The drawing under review shows one solid part. Ordinate dimensions are in mm from its lowest x, y, z. Give positions to 0.01 mm unless a question says otherwise; leave off trailing zeros. Loops run counter-clockwise (first coordinate to the right, second up) from the corner with the lowest first, then second, coordinate; pieces in that order, holes last. Notation, with made-up numbers: M 18,75.5 L 65,75.5 A18 cw 65,89.5 Z; hole C -13,-6.5 d4. An arc over 180 degrees is marked long. Write item = value, one per line. Start each with the question number.
1. For pin 1 (2 mm diameter, centred on y = 4, z = 7, fed in from -X), flat-tipped, find the tip position at first contact; note if it passes through.
2. We need section D-D on y = 4.2. Give the boundary of the cut face in (x, z).
3. Wall thickness on line 1 along Z through (x, y) = (80, 2.55); line 2 along X through (y, z) = (3.05, 10); line 3 along Z through (x, y) = (49, 2.35): over which ranges is each line inside the solid? List them lowest first. Write a range as from..to.
4. We need section A-A on x = 50. Give the boundary of the cut face in (y, z).
5. We need section B-B on z = 13.8. Give the boundary of the cut face in (x, y), then the cut area to 3 significant figures.
6. We need section C-C on x = 25. Give the boundary of the cut face in (y, z).
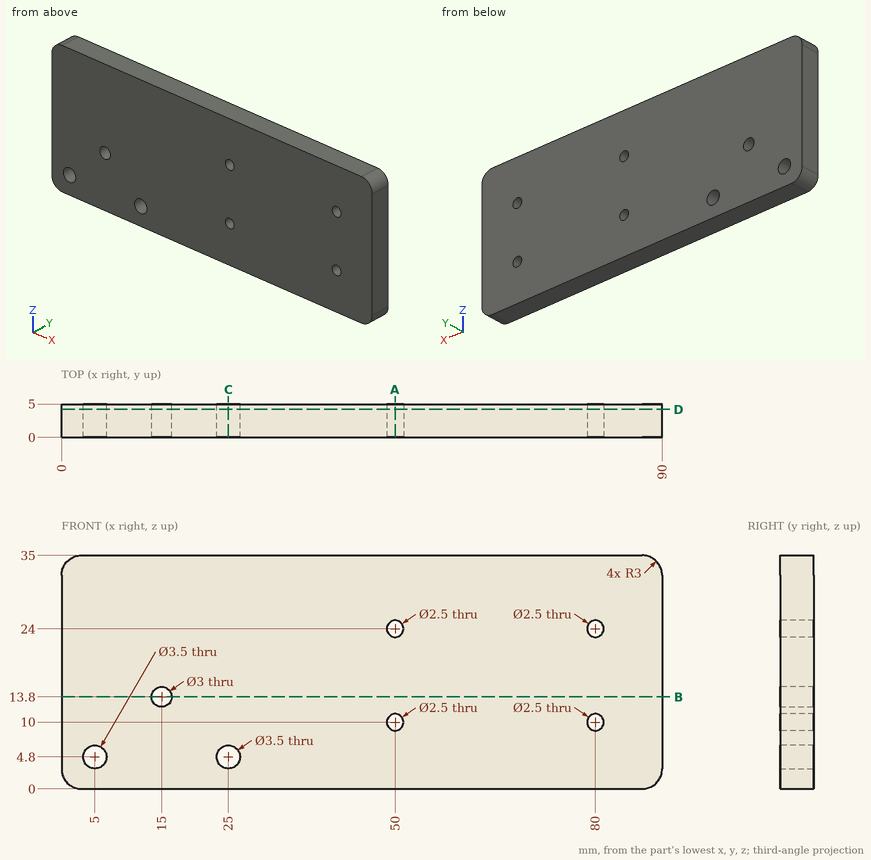
Final values:
q1.pin_1 = 0
q2.outline = M 0,3 A3 ccw 3,0 L 87,0 A3 ccw 90,3 L 90,32 A3 ccw 87,35 L 3,35 A3 ccw 0,32 Z; hole C 5,4.8 d3.5; hole C 15,13.8 d3; hole C 25,4.8 d3.5; hole C 50,10 d2.5; hole C 50,24 d2.5; hole C 80,10 d2.5; hole C 80,24 d2.5
q3.line_1 = 0..8.75, 11.25..22.75, 25.25..35
q3.line_2 = 0..48.75, 51.25..78.75, 81.25..90
q3.line_3 = 0..9.25, 10.75..23.25, 24.75..35
q4.outline = M 0,0 L 5,0 L 5,8.75 L 0,8.75 Z; M 0,11.25 L 5,11.25 L 5,22.75 L 0,22.75 Z; M 0,25.25 L 5,25.25 L 5,35 L 0,35 Z
q5.outline = M 0,0 L 13.5,0 L 13.5,5 L 0,5 Z; M 16.5,0 L 90,0 L 90,5 L 16.5,5 Z
q5.area = 435 mm²
q6.outline = M 0,0 L 5,0 L 5,3.05 L 0,3.05 Z; M 0,6.55 L 5,6.55 L 5,35 L 0,35 Z
